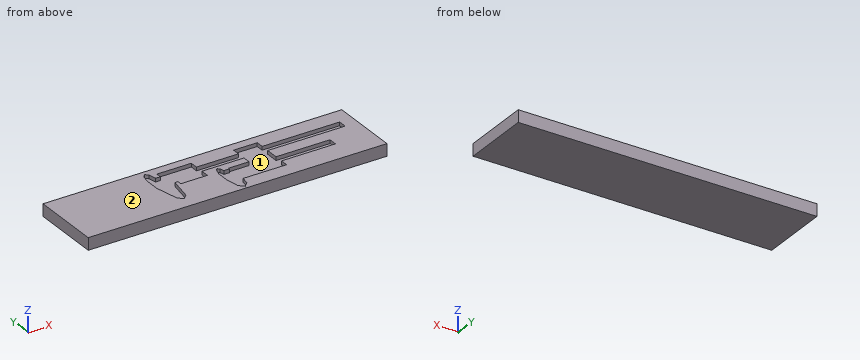
```python
from build123d import *

# Parameters (mm, degrees)
F0_W     = 625.475
F0_H     = 146.05
F3_DEPTH = 25.4
F4_DEPTH = 7.62
F2_W     = 49.53
F2_H     = 17.78
F2_H_2   = 16.2543391211
F2_W_2   = 162.1558675107
F2_H_3   = 15.875
F5_DEPTH = 7.62


with BuildPart() as f3:
    # F0 (on Top) → F3 (new body)
    with BuildSketch(Plane.XY):
        Rectangle(F0_W, F0_H)
    extrude(amount=-F3_DEPTH)

    # F1 (on Top) → F4 (cut)
    with BuildSketch(Plane.XY):
        Polygon((5.1413444427, -28.5038674987), (10.2213444427, -57.7138674987), (19.7463444427, -67.2388674987), (29.2713444427, -57.7138674987), (32.1426487905, -41.2038674987), (123.2513444427, -41.2038674987), (123.2513444427, -24.6938674987), (236.2813444427, -24.6938674987), (236.2813444427, -6.9138674987), (123.2513444427, -6.9138674987), (123.2513444427, 3.7541325013), (30.5413444427, 3.7541325013), (30.5413444427, 0.7061325013), (30.5413444427, -4.3738674987), (20.3813444427, -4.3738674987), (19.0962397041, 0.7061325013), (16.8448203131, 9.6059600121), (12.7613444427, 13.4061325013), (9.2248203131, 9.6059600121), (5.1413444427, -4.3738674987), align=None)
        Polygon((30.5413444427, 0.7061325013), (19.0962397041, 0.7061325013), (20.3813444427, -4.3738674987), (30.5413444427, -4.3738674987), align=None)
    extrude(amount=-F4_DEPTH, mode=Mode.SUBTRACT)

    # F2 (on Top) → F5 (cut)
    with BuildSketch(Plane.XY):
        Polygon((-114.6427880466, 11.1184716225), (-104.0148213506, -37.1415283775), (-94.4898213506, -46.6665283775), (-84.9648213506, -37.1415283775), (-76.5427880466, 11.1184716225), (-70.1927880466, 11.1184716225), (-70.1927880466, 2.2284716225), (-14.3127880466, 2.2284716225), (-14.3127880466, 20.0084716225), (73.7213444427, 20.0084716225), (73.7213444427, 37.7884716225), (-14.3127880466, 37.7884716225), (-14.3127880466, 54.2984716225), (-86.7027880466, 54.2984716225), (-86.7027880466, 42.8684716225), (-96.8627880466, 42.8684716225), (-99.627574241, 58.7582128885), (-105.7527880466, 64.4584716225), (-111.057574241, 58.7582128885), (-114.6427880466, 42.8684716225), align=None)
        with Locations((98.4863444427, 28.8984716225)):
            Rectangle(F2_W, F2_H)
        with Locations((98.4863444427, 11.8813020619)):
            Rectangle(F2_W, F2_H_2)
        with Locations((204.329278198, 28.8984716225)):
            Rectangle(F2_W_2, F2_H)
        with Locations((98.4863444427, 45.7259716225)):
            Rectangle(F2_W, F2_H_3)
    extrude(amount=-F5_DEPTH, mode=Mode.SUBTRACT)


solid = f3.part
```
Read the model definition and answer for the solid it produces. Units are mm, in the model's axes. Face numbers are marked on the shaded views. Round coordinates to 2 decimals unless told otherwise and drop trailing zeros. Write each loop counter-clockwise with the first axis right and the second up, starting at its lowest first coordinate (ties: lowest second). Pieces come first, ordered by that corner, then holes. Notation, with made-up numbers: (19.5, -4.75) - (35.5, -4.75) arc R21 cw to (35.5, 9.25) - close; hole circle Ø10 at (89.5, 72). An arc over 180 degrees is marked (long way). One line per item, written item: value.
Q1. For a pull along Y with two mould halves and no side action, classify the marked faces 1 and 2 as pulls with the +Y half, pulls with the -Y half, needs draft (parallel to the pull), parting line crosses it, or undercut.
The answers:
face 1: undercut
face 2: needs draft
Q2. Straight lines are drawn through the part: line 1 (Y direction, x = 117, z = -6) (3 decimals); line 2 (Y direction, x = -43, z = -6) (3 decimals); line 3 (X direction, y = 22, z = -5.25). For each, find the intervals that lie inside material, in ascending order. Write a range as from..to.
The answers:
line 1: y = -73.025..-41.204, 53.663..73.025
line 2: y = -73.025..2.228, 54.298..73.025
line 3: x = -312.74..-114.64, 285.41..312.74
Q3. Find section C-C (x = -30). Determine the outline of the cut face in (y, z) (3 decimals).
The answers:
outline: (-73.025, -25.4) - (73.025, -25.4) - (73.025, 0) - (54.298, 0) - (54.298, -7.62) - (2.228, -7.62) - (2.228, 0) - (-73.025, 0) - close
Q4. Find section B-B (x = 110). Determine the outline of the cut face in (y, z) (3 decimals).
The answers:
outline: (-73.025, -25.4) - (73.025, -25.4) - (73.025, 0) - (53.663, 0) - (53.663, -7.62) - (-41.204, -7.62) - (-41.204, 0) - (-73.025, 0) - close
Q5. Find section A-A (x = 185). Determine the outline of the cut face in (y, z) (3 decimals), and give its area (3 significant figures).
The answers:
outline: (-73.025, -25.4) - (73.025, -25.4) - (73.025, 0) - (37.788, 0) - (37.788, -7.62) - (20.008, -7.62) - (20.008, 0) - (-6.914, 0) - (-6.914, -7.62) - (-24.694, -7.62) - (-24.694, 0) - (-73.025, 0) - close
area: 3,440 mm2
